Here's how the part is built. I have some questions about the finished solid (model axes, mm). Face numbers are marked on the shaded views. Coordinates: 2 decimals unless noted, no trailing zeros. Write each loop counter-clockwise with the first axis right and the second up, starting at its lowest first coordinate (ties: lowest second). Pieces come first, ordered by that corner, then holes. Notation, with made-up numbers: M -11.75,77.25 L 39.25,77.25 A28 cw 39.25,110.25 Z; hole C -12,-24 d5. An arc over 180 degrees is marked long. Use one line per item in the form item = value. Start each with the question number.
1. Thinking about a two-plate mould opening in X: for the marked faces 1, 2 and 3, which applies, released by +X, released by -X, zero draft, split by the parting line, or undercut?
2. I want a section at B-B, the plane z = 1.25. List the corners of the cut face in (x, y) for me.
3. I want a section at C-C, the plane x = 5.25. List the corners of the cut face in (y, z) for me, plus the area to 3 significant figures.
4. I want a section at A-A, the plane y = 3. List the corners of the cut face in (x, z) for me.
5. I want a section at D-D, the plane x = 1.25. List the corners of the cut face in (y, z) for me, plus the area to 3 significant figures.
6. Please list where these lines run through material, in increasing order: line 1 along Y through (x, z) = (5, 1.5); line 2 along X through (y, z) = (25, 1.05); line 3 along Y through (x, z) = (6, 0.4). Write a range as [from, to].
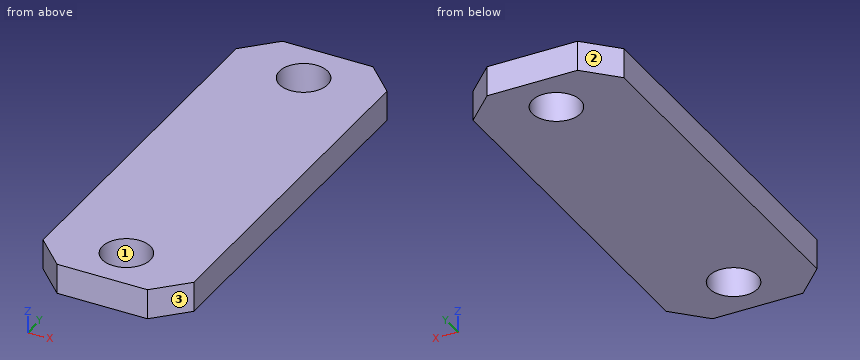
Autodesk Inventor part; units mm, degrees
ref_plane "YZ Plane" through (0, 0, 0) normal (1, 0, 0) x (0, 1, 0)
ref_plane "XZ Plane" through (0, 0, 0) normal (0, 1, 0) x (-1, 0, 0)
ref_plane "XY Plane" through (0, 0, 0) normal (0, 0, 1) x (1, 0, 0)
sketch "スケッチ1" plane through (0, 0, 0) normal (0, 0, 1) x (1, 0, 0)
  line L0 (0, 0) -> (10, 0)
  line L1 (10, 0) -> (10, 28)
  line L2 (10, 28) -> (0, 28)
  line L3 (0, 28) -> (0, 0)
  dimension "d0" = 10
  dimension "d1" = 28
extrude "押し出し1" add sketch "スケッチ1" along normal blind 2
sketch "スケッチ2" plane through (0, 0, 2) normal (0, 0, 1) x (1, 0, 0)
  line L0 (10, 28) -> (0, 28)
  line L1 (10, 0) -> (10, 28)
  line L2 (0, 0) -> (10, 0)
  point P0 (5, 3)
  dimension "d6" = 5
  dimension "d7" = 3
hole "穴1" at (5, 3, 2) direction (0, 0, -1) diameter 3.2 end through all
sketch "スケッチ7" plane through (0, 0, 2) normal (0, 0, 1) x (1, 0, 0)
  line L0 (10, 0) -> (10, 28)
  line L1 (10, 28) -> (0, 28)
  point P0 (0, 0)
  point P1 (5, 25)
  point P2 (6, 3)
  point P3 (6, 27)
  point P4 (5, 28)
  point P5 (1, 28)
  point P6 (6, 2)
  dimension "d43" = 5
  dimension "d44" = 3
hole "穴2" at (5, 25, 2) direction (0, 0, -1) diameter 3.2 end through all
sketch "スケッチ8" plane through (0, 0, 2) normal (0, 0, 1) x (1, 0, 0)
  line L0 (10, 28) -> (0, 28)
  line L1 (8, 28) -> (10, 26)
  line L2 (10, 0) -> (10, 28)
  line L3 (0, 28) -> (0, 0)
  line L4 (0, 26) -> (2, 28)
  line L5 (0, 0) -> (10, 0)
  line L6 (2, 0) -> (0, 2)
  line L7 (8, 0) -> (10, 2)
  dimension "d45" = 2
  dimension "d46" = 2
  dimension "d49" = 2
  dimension "d50" = 2
  dimension "d51" = 2
  dimension "d52" = 2
  dimension "d53" = 2
  dimension "d54" = 2
extrude "押し出し5" cut sketch "スケッチ8" against normal blind 10 contours L2 L1 L0 | L4 L3 L0 | L2 L5 L7 | L6 L5 L3
properties part number "リンク26×6×2"
Answer list:
q1.face_1 = undercut
q1.face_2 = released by -X
q1.face_3 = released by +X
q2.outline = M 0,2 L 2,0 L 8,0 L 10,2 L 10,26 L 8,28 L 2,28 L 0,26 Z; hole C 5,3 d3.2; hole C 5,25 d3.2
q3.outline = M 0,0 L 1.42,0 L 1.42,2 L 0,2 Z; M 4.58,0 L 23.42,0 L 23.42,2 L 4.58,2 Z; M 26.58,0 L 28,0 L 28,2 L 26.58,2 Z
q3.area = 43.4 mm²
q4.outline = M 0,0 L 3.4,0 L 3.4,2 L 0,2 Z; M 6.6,0 L 10,0 L 10,2 L 6.6,2 Z
q5.outline = M 0.75,0 L 27.25,0 L 27.25,2 L 0.75,2 Z
q5.area = 53.0 mm²
q6.line_1 = [0, 1.4], [4.6, 23.4], [26.6, 28]
q6.line_2 = [0, 3.4], [6.6, 10]
q6.line_3 = [0, 1.75], [4.25, 23.75], [26.25, 28]
